Build history of the part. All positions in model axes, mm. A direction names the side the tool comes from. Round coordinates to 2 decimals unless told otherwise and drop trailing zeros. Write each loop counter-clockwise with the first axis right and the second up, starting at its lowest first coordinate (ties: lowest second). Pieces come first, ordered by that corner, then holes. Notation, with made-up numbers: (18.25, -15.75) -> (31.25, -15.75) arc R18 ccw to (31.25, -0.75) -> close; hole circle Ø3 at (87.25, 61). An arc over 180 degrees is marked (long way). Answer in a Markdown table with one row per item.
```python
from build123d import *

# Parameters (mm, degrees)
BOSS_EXTRUDE1_DEPTH = 12
BOSS_EXTRUDE2_DEPTH = 12
CHAMFER1_SIZE       = 12
SKETCH3_R           = 12
CUT_EXTRUDE1_DEPTH  = 132.554171352


with BuildPart() as part:
    # Sketch1 → Boss-Extrude1 (new body)
    with BuildSketch(Plane.XY):
        with BuildLine():
            Line((0, 37.5), (70, 37.5))
            ThreePointArc((70, 37.5), (107.5, 0), (70, -37.5))
            Line((70, -37.5), (0, -37.5))
            ThreePointArc((0, -37.5), (-37.5, 0), (0, 37.5))
        make_face()
    extrude(amount=BOSS_EXTRUDE1_DEPTH)

    # Sketch2 → Boss-Extrude2 (add)
    with BuildSketch(Plane(origin=(0, 0, 0), x_dir=(-1, 0, 0), z_dir=(0, 0, -1))):
        with BuildLine():
            Line((0, -49.5), (-70, -49.5))
            ThreePointArc((-70, -49.5), (-119.5, 0), (-70, 49.5))
            Line((-70, 49.5), (0, 49.5))
            ThreePointArc((0, 49.5), (49.5, 0), (0, -49.5))
        make_face()
    extrude(amount=BOSS_EXTRUDE2_DEPTH)

    # Chamfer1
    chamfer1_edges = [part.edges().sort_by_distance(p)[0] for p in [
        (35, 49.5, 0),
        (119.5, 0, 0),
        (35, -49.5, 0),
        (-49.5, 0, 0),
    ]]
    chamfer(chamfer1_edges, length=CHAMFER1_SIZE - 0.0001)  # a hair under: the kernel refuses the full size

    # Sketch3 → Cut-Extrude1 (cut, through all)
    with BuildSketch(Plane.XY.offset(12)):
        Circle(SKETCH3_R)
        with Locations((70, 0)):
            Circle(SKETCH3_R)
    extrude(amount=-CUT_EXTRUDE1_DEPTH, mode=Mode.SUBTRACT)


solid = part.part
```
Q1. Two-plate mould, pull along X, no slides. Class faces 1 (the flat face through (35.5, 43.6, -6.1)), 2 (the cylindrical face through (60.477, -7.302, 0.168)), 3 (the conical face through (108.24, -0.84, -0.75)), 4 (the conical face through (-38.24, 0.84, -0.75)): released by +X, released by -X, zero draft, split by the parting line, or undercut.
A:
| item | result |
|---|---|
| face 1 | zero draft |
| face 2 | undercut |
| face 3 | released by +X |
| face 4 | released by -X |
Q2. Saw through at A-A on y = 0. State how many separate pieces and enclosed holes the cut face has, plus the area to 3 significant figures.
A:
| item | result |
|---|---|
| separate pieces | 3 |
| enclosed holes | 0 |
| area | 2,470 mm² |
Q3. Which spindle directions (+Z, -Z, +X, -X, +Y, -Y) get a long thin tool onto all of the face, cutting with end or side? Do faces 5 (the flat face through (35, -37.5, 6)), 6 (the cylindrical face through (-37.49, -0.82, 5.92)), 7 (the flat face through (35, 37.5, 6)). Say none if no direction does.
A:
| item | result |
|---|---|
| face 5 | +Z, +X, -X, -Y |
| face 6 | +Z, -X |
| face 7 | +Z, +X, -X, +Y |
Q4. Wall check: line 1 (Y direction, x = 0, z = 1.75); line 2 (X direction, y = 3, z = 3.75); line 3 (X direction, y = 1, z = -10). Give the ranges that are in metal, low to high. Write a range as [from, to].
A:
| item | result |
|---|---|
| line 1 | [-37.5, -12], [12, 37.5] |
| line 2 | [-37.38, -11.62], [11.62, 58.38], [81.62, 107.38] |
| line 3 | [-47.49, -11.96], [11.96, 58.04], [81.96, 117.49] |
Q5. Saw through at B-B on z = 4. Write the cut outline in (x, y), plus the area to 3 significant figures.
A:
| item | result |
|---|---|
| outline | (0, -37.5) -> (70, -37.5) arc R37.5 ccw to (70, 37.5) -> (0, 37.5) arc R37.5 ccw to start; hole circle Ø24 at (0, 0); hole circle Ø24 at (70, 0) |
| area | 8,760 mm² |
Q6. Drop flat-ended pins along their axis: P1, Ø19, axis at x = 70, y = 0, coming from the -Z side; P2, Ø8, axis at y = 8.5, z = -7.5, coming from the -X side; P3, Ø1.5, axis at x = 69, z = -7.5, coming from the -Y side; P4, Ø2, axis at y = -16, z = 8.5, coming from the +X side. Give the stop position or say it passes through.
A:
| item | result |
|---|---|
| P1 | through |
| P2 | x = -48.31 |
| P3 | y = -45.75 |
| P4 | x = 104.37 |
